Autodesk Fusion 360 part; units mm, degrees
sketch "Sketch1" plane through (0, 0, 0) normal (0, 0, 1) x (1, 0, 0) in component "2.4\" LCD Module"
  line L0 (0, 0) -> (71, 0)
  line L1 (71, 0) -> (71, 43.3)
  line L2 (71, 43.3) -> (0, 43.3)
  line L3 (0, 43.3) -> (0, 0)
  dimension "d1" = 71
  dimension "d2" = 43.3
extrude "Extrude1" add sketch "Sketch1" along normal blind 1.7 in component "2.4\" LCD Module"
hole "Hole1" at (68.5, 2.5, 1.7) direction (0, 0, -1) diameter 3 depth 5 tip angle 180 in component "2.4\" LCD Module"
hole "Hole2" at (68.5, 40.8, 1.7) direction (0, 0, -1) diameter 3 depth 5 tip angle 180 in component "2.4\" LCD Module"
hole "Hole3" at (2.5, 2.5, 1.7) direction (0, 0, -1) diameter 3 depth 5 tip angle 180 in component "2.4\" LCD Module"
hole "Hole4" at (2.5, 40.8, 1.7) direction (0, 0, -1) diameter 3 depth 5 tip angle 180 in component "2.4\" LCD Module"
fillet "Fillet1" radius 3 4 edges at (71, 0, 0.85) (0, 0, 0.85) (71, 43.3, 0.85) (0, 43.3, 0.85) in component "2.4\" LCD Module"
sketch "Sketch2" plane through (0, 0, 1.7) normal (0, 0, 1) x (-1, 0, 0) in component "2.4\" LCD Module"
  arc A0 (-3, -43.3) -> (0, -40.3) centre (-3, -40.3) ccw
  line L0 (0, -40.3) -> (0, -3)
  arc A1 (0, -3) -> (-3, 0) centre (-3, -3) ccw
  line L1 (-3, 0) -> (-68, 0)
  arc A2 (-68, 0) -> (-71, -3) centre (-68, -3) ccw
  line L2 (-71, -3) -> (-71, -40.3)
  arc A3 (-71, -40.3) -> (-68, -43.3) centre (-68, -40.3) ccw
  line L3 (-68, -43.3) -> (-3, -43.3)
  circle A4 centre (-2.5, -40.8) radius 1.5
  circle A5 centre (-2.5, -2.5) radius 1.5
  circle A6 centre (-68.5, -40.8) radius 1.5
  circle A7 centre (-68.5, -2.5) radius 1.5
  line L4 (-5.4496, 0.0416) -> (-65.5496, 0.0416)
  line L5 (-65.5496, 0.0416) -> (-65.5496, -43.2584)
  line L6 (-65.5496, -43.2584) -> (-5.4496, -43.2584)
  line L7 (-5.4496, -43.2584) -> (-5.4496, 0.0416)
  line L8 (-5.4496, 0.0416) -> (-65.5496, -43.2584) construction
  line L9 (-65.5496, 0.0416) -> (-5.4496, -43.2584) construction
  point P0 (-35.4996, -21.6084)
  dimension "d27" = 60.1
  dimension "d28" = 43.3
extrude "Extrude2" add sketch "Sketch2" along normal blind 2.45 contours L1 L5 L6 L7 in component "2.4\" LCD Module"
sketch "Sketch3" plane through (0, 0, 1.7) normal (0, 0, 1) x (-1, 0, 0) in component "2.4\" LCD Module"
  line L0 (-65.5496, -43.2584) -> (-65.5496, 0)
  line L1 (-65.5496, 0) -> (-68, 0)
  arc A0 (-68, 0) -> (-71, -3) centre (-68, -3) ccw
  line L2 (-71, -3) -> (-71, -40.3)
  arc A1 (-71, -40.3) -> (-68, -43.3) centre (-68, -40.3) ccw
  line L3 (-68, -43.3) -> (-3, -43.3)
  arc A2 (-3, -43.3) -> (0, -40.3) centre (-3, -40.3) ccw
  line L4 (0, -40.3) -> (0, -3)
  arc A3 (0, -3) -> (-3, 0) centre (-3, -3) ccw
  line L5 (-3, 0) -> (-5.4496, 0)
  line L6 (-5.4496, 0) -> (-5.4496, -43.2584)
  line L7 (-5.4496, -43.2584) -> (-65.5496, -43.2584)
  circle A4 centre (-2.5, -40.8) radius 1.5
  circle A5 centre (-2.5, -2.5) radius 1.5
  circle A6 centre (-68.5, -40.8) radius 1.5
  circle A7 centre (-68.5, -2.5) radius 1.5
  point P0 (-68.5, -12.7999)
  point P1 (-68.5, -15.3285)
  point P2 (-68.5, -17.857)
  point P3 (-68.5, -20.3856)
  point P4 (-68.5, -22.9142)
  point P5 (-68.5, -25.4427)
  point P6 (-68.5, -27.9713)
  point P7 (-68.5, -30.4999)
  dimension "d33" = 17.7
  dimension "d34" = 0
hole "Hole5" at (68.5, 12.7999, 1.7) at (68.5, 15.3285, 1.7) at (68.5, 17.857, 1.7) at (68.5, 20.3856, 1.7) at (68.5, 22.9142, 1.7) at (68.5, 25.4427, 1.7) at (68.5, 27.9713, 1.7) at (68.5, 30.4999, 1.7) direction (0, 0, -1) diameter 1 depth 5 tip angle 180 in component "2.4\" LCD Module"
sketch "Sketch4" plane through (0, 0, 0) normal (0, 0, -1) x (1, 0, 0) in component "2.4\" LCD Module"
  circle A0 centre (68.5, -27.9713) radius 0.5
  circle A1 centre (68.5, -22.9142) radius 0.5
  circle A2 centre (68.5, -17.857) radius 0.5
  circle A3 centre (68.5, -12.7999) radius 0.5
  circle A4 centre (68.5, -15.3285) radius 0.5
  circle A5 centre (68.5, -20.3856) radius 0.5
  circle A6 centre (68.5, -25.4427) radius 0.5
  circle A7 centre (68.5, -30.4999) radius 0.5
  circle A8 centre (2.5, -40.8) radius 1.5
  circle A9 centre (2.5, -2.5) radius 1.5
  circle A10 centre (68.5, -40.8) radius 1.5
  circle A11 centre (68.5, -2.5) radius 1.5
  arc A12 (0, -40.3) -> (3, -43.3) centre (3, -40.3) ccw
  line L0 (3, -43.3) -> (68, -43.3)
  arc A13 (68, -43.3) -> (71, -40.3) centre (68, -40.3) ccw
  line L1 (71, -40.3) -> (71, -3)
  arc A14 (71, -3) -> (68, 0) centre (68, -3) ccw
  line L2 (68, 0) -> (3, 0)
  arc A15 (3, 0) -> (0, -3) centre (3, -3) ccw
  line L3 (0, -3) -> (0, -40.3)
  line L4 (12.6, -31.65) -> (5, -31.65)
  line L5 (5, -31.65) -> (5, -11.65)
  line L6 (5, -11.65) -> (12.6, -11.65)
  line L7 (12.6, -11.65) -> (12.6, -31.65)
  dimension "d38" = 7.6
  dimension "d39" = 20
extrude "Extrude3" add sketch "Sketch4" along normal blind 5.52 contours L4 L5 L6 L7 in component "2.4\" LCD Module"
component "2.4\" LCD Module" placed x (1, 0, 0) y (0, 1, 0) z (0, 0, 1) at (0, 0, 0)
Read the model definition and answer for the solid it produces. Units are mm, in the model's axes. A direction names the side the tool comes from. Coordinates: 2 decimals unless noted, no trailing zeros. Order: outer loops, then holes, each group sorted by start corner. A loop starts at its lowest first (then second) coordinate and runs counter-clockwise, first axis right, second up. Notation, with made-up numbers: M 67.25,-5.75 L 117.25,-5.75 A14 ccw 117.25,8.25 Z; hole C 68.25,-28.5 d5. An arc over 180 degrees is marked long. Put each result on its own line as item: value. Start each with the question number.
Item 1: Section C-C, the plane z = -3.5 is taken. Determine the outline of the cut face in (x, y).
Item 2: Section A-A, the plane y = 8 is taken. Determine the outline of the cut face in (x, z).
Item 3: Section B-B, the plane x = 26 is taken. Determine the outline of the cut face in (y, z).
Item 4: For faces 4 (the face through (5, 22, -3)), 5 (the face through (5.45, 22, 3)), 6 (the face through (9, 11.65, -3)), determine the directions among +Z, -Z, +X, -X, +Y, -Y from which every point of the face is accessible in a straight line to the end or side of a thin tool.
Item 5: Consider probe 1 along X at (y, z) = (40.8, 0.55); probe 2 along X at (y, z) = (2, 2.5); probe 3 along Y at (x, z) = (2.5, 0.65). Determine where each line is inside the solid, lowest interval first. Write a range as [from, to].
Item 6: The mould has two halves that part along Y. Classify faces 1 (the face through (67.235, 1.694, 0.838)), 2 (the face through (4, 22, 1.7)), 3 (the face through (36, 43.258, 3)): +Y half, -Y half, draft (parallel to the pull), parting line (faces both ways), or undercut.
Item 7: Given pin 1 Ø2 at (x, y) = (46.5, 9.5) entering from -Z; pin 2 Ø3.5 at (x, y) = (2.5, 40.8) entering from +Z; pin 3 Ø1.7 at (y, z) = (18, -3.5) entering from +X; pin 4 Ø3 at (x, z) = (29, -2.5) entering from -Y, each flat-ended and moving along its own axis, determine where each tip first touches the part or whether it passes through.
Computed:
1. outline: M 5,11.65 L 12.6,11.65 L 12.6,31.65 L 5,31.65 Z
2. outline: M 0,0 L 71,0 L 71,1.7 L 65.55,1.7 L 65.55,4.15 L 5.45,4.15 L 5.45,1.7 L 0,1.7 Z
3. outline: M 0,0 L 43.3,0 L 43.3,1.7 L 43.26,1.7 L 43.26,4.15 L 0,4.15 Z
4. face 4: -Z, -X, +Y, -Y
4. face 5: +Z, -X, +Y, -Y
4. face 6: -Z, +X, -X, -Y
5. probe 1: x = [0.04, 1], [4, 67], [70, 70.96]
5. probe 2: x = [5.45, 65.55]
5. probe 3: y = [0.04, 1], [4, 39.3], [42.3, 43.26]
6. face 1: undercut
6. face 2: draft
6. face 3: +Y half
7. pin 1: stops at z = 0
7. pin 2: stops at z = 1.7
7. pin 3: stops at x = 12.6
7. pin 4: passes through
